from build123d import *

# Parameters (mm, degrees)
IZIM2_W                     = 150
IZIM2_H                     = 7
IZIM2_W_2                   = 130
IZIM2_H_2                   = 80
IZIM3_R                     = 127
Y_KSEKLIK_EKSTR_ZYON1_DEPTH = 2
RADYUS1_R                   = 1
RADYUS2_R                   = 1
IZIM5_R                     = 55
Y_KSEKLIK_EKSTR_ZYON2_DEPTH = 6


with BuildPart() as part:
    # Çizim2 → Döndür1 (revolve)
    with BuildSketch(Plane.XY, mode=Mode.PRIVATE) as d_nd_r1_sk:
        with Locations((-75, 3.5)):
            Rectangle(IZIM2_W, IZIM2_H)
        with Locations((-65, 47)):
            Rectangle(IZIM2_W_2, IZIM2_H_2)
    revolve(d_nd_r1_sk.sketch.rotate(Axis((0, 7, 0), (0, 1, 0)), 270), axis=Axis((0, 7, 0), (0, 1, 0)))

    # Çizim3 → Yükseklik-Ekstrüzyon1 (add)
    with BuildSketch(Plane(origin=(0, 87, 0), x_dir=(1, 0, 0), z_dir=(0, 1, 0))):
        with Locations(Location((0, 0, 0), (0, 0, 270))):
            Circle(IZIM3_R)
    extrude(amount=Y_KSEKLIK_EKSTR_ZYON1_DEPTH)

    # Radyus1
    radyus1_edges = [part.edges().sort_by_distance(p)[0] for p in [
        (0, 87, 130),
        (0, 7, 130),
    ]]
    fillet(radyus1_edges, radius=RADYUS1_R)

    # Radyus2
    radyus2_edges = [part.edges().sort_by_distance(p)[0] for p in [
        (0, 7, 150),
    ]]
    fillet(radyus2_edges, radius=RADYUS2_R)

    # Çizim5 → Yükseklik-Ekstrüzyon2 (add)
    with BuildSketch(Plane(origin=(0, 89, 0), x_dir=(1, 0, 0), z_dir=(0, 1, 0))):
        with Locations(Location((0, 0, 0), (0, 0, 270))):
            Circle(IZIM5_R)
    extrude(amount=Y_KSEKLIK_EKSTR_ZYON2_DEPTH)


solid = part.part
Source: CAD feature listing. Evaluate the final solid. Frame: model axes, mm. A direction names the side the tool comes from. Round coordinates to 2 decimals unless told otherwise and drop trailing zeros. Order: outer loops, then holes, each group sorted by start corner. A loop starts at its lowest first (then second) coordinate and runs counter-clockwise, first axis right, second up. Notation, with made-up numbers: (57.25, 84) -> (97.25, 84) arc R10 cw to (97.25, 99) -> close; hole circle Ø6 at (29.5, 85). An arc over 180 degrees is marked (long way). Answer as CSV lines item,"result".
Item 1: Line query: L1, parallel to Y at x = -26.5, z = 116.5; L2, parallel to Y at x = 128, z = 70; L3, parallel to X at y = 28, z = 114.5. Output: solid intervals per line, ascending.
A:
L1,"0 to 89"
L2,"0 to 7"
L3,"-61.56 to 61.56"
Item 2: Reachability of faces 1 (the face through (-48.794, 91.958, 25.379)), 2 (the face through (-2, 0, 2)) from +Z, -Z, +X, -X, +Y, -Y: full face, straight path, thin tool, end or side. Return the list, or none.
A:
face 1,"+Y"
face 2,"+Z, -Z, +X, -X, -Y"
Item 3: Pin query (flat end, axial travel): pin 1 Ø2 at (y, z) = (68.5, -60) entering from +X; pin 2 Ø3 at (y, z) = (80, 74) entering from +X; pin 3 Ø10 at (y, z) = (44, 86.5) entering from +X. Return the tip coordinate at first contact, or that it passes through.
A:
pin 1,"x = 115.84"
pin 2,"x = 107.91"
pin 3,"x = 101.28"
Item 4: Section C-C, the plane y = 14. Return loops of the section in (x, z), plus the area to 3 significant figures.
A:
outline,"circle Ø260 at (0, 0)"
area,"53,100 mm²"
Item 5: Section A-A, the plane z = 0. Return loops of the section in (x, y).
A:
outline,"(-150, 0) -> (150, 0) -> (150, 6) arc R1 ccw to (149, 7) -> (131, 7) arc R1 cw to (130, 8) -> (130, 86) arc R1 ccw to (129, 87) -> (127, 87) -> (127, 89) -> (55, 89) -> (55, 95) -> (-55, 95) -> (-55, 89) -> (-127, 89) -> (-127, 87) -> (-129, 87) arc R1 ccw to (-130, 86) -> (-130, 8) arc R1 cw to (-131, 7) -> (-149, 7) arc R1 ccw to (-150, 6) -> close"
Item 6: Section B-B, the plane x = 0. Return loops of the section in (y, z), plus the area to 3 significant figures.
A:
outline,"(0, -150) -> (6, -150) arc R1 ccw to (7, -149) -> (7, -131) arc R1 cw to (8, -130) -> (86, -130) arc R1 ccw to (87, -129) -> (87, -127) -> (89, -127) -> (89, -55) -> (95, -55) -> (95, 55) -> (89, 55) -> (89, 127) -> (87, 127) -> (87, 129) arc R1 ccw to (86, 130) -> (8, 130) arc R1 cw to (7, 131) -> (7, 149) arc R1 ccw to (6, 150) -> (0, 150) -> close"
area,"24,100 mm²"
